Part print with two shaded views. Sizes in mm from the minimum x, y, z corner. Coordinates: 2 decimals unless noted, no trailing zeros. Loops run counter-clockwise (first coordinate to the right, second up) from the corner with the lowest first, then second, coordinate; pieces in that order, holes last.
(1) Slice it at B-B (z = 0.5). Give the cut face in (x, y).
(2) Slice it at A-A (x = 5.5). Give the cut face in (y, z), and give its area (3 significant figures).
(3) Flat gauge pin, fed straight in: P1, Ø0.6, axis at x = 0.5, z = 4.5, coming from the +Y side. Where does the tip first touch, or does it go through?
(4) Slice it at D-D (z = 2.5). Give the cut face in (x, y).
(5) Wall check: L1, parallel to Z at x = 5.75, y = 0.1; L2, parallel to X at y = 0.7, z = 1.6; L3, parallel to X at y = 0.6, z = 4.5. Give the ranges that are in metal, low to high.
(6) Slice it at C-C (y = 0.25). Give the cut face in (x, z).
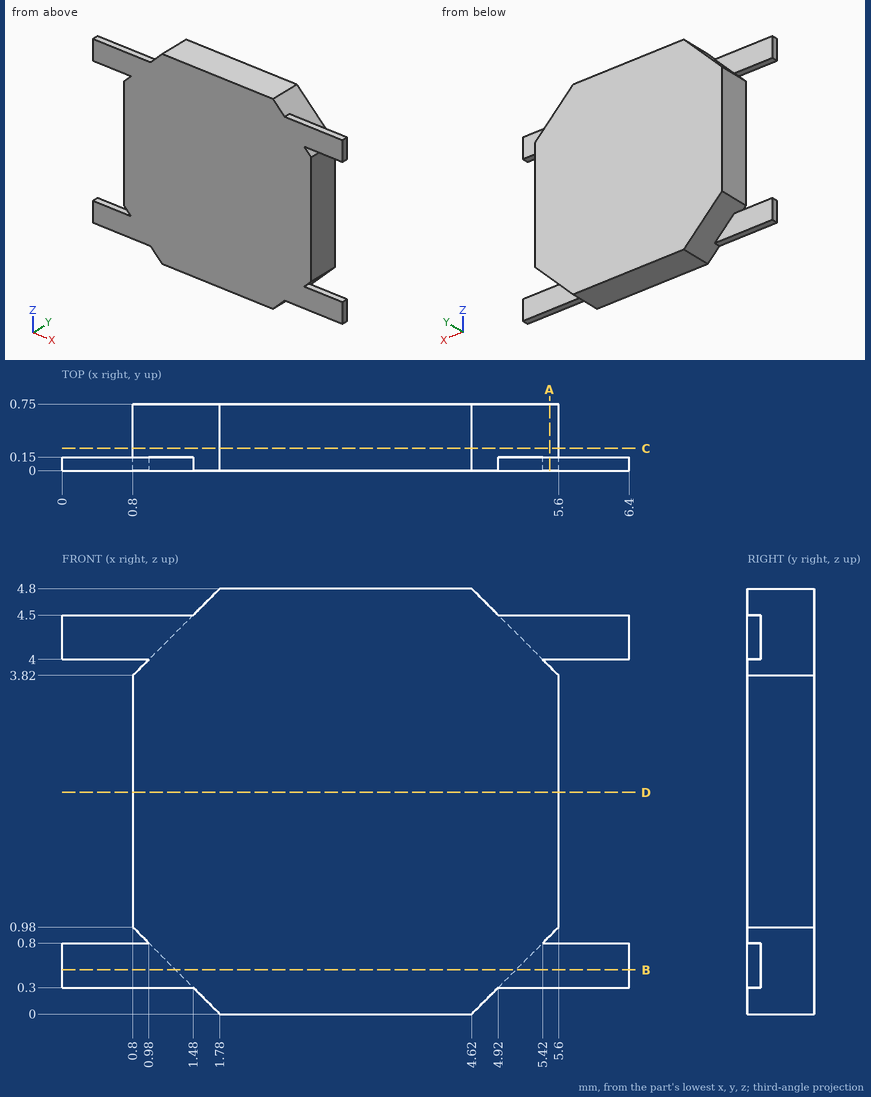
Response values:
1. outline: (0, 0) - (6.4, 0) - (6.4, 0.15) - (5.12, 0.15) - (5.12, 0.75) - (1.28, 0.75) - (1.28, 0.15) - (0, 0.15) - close
2. outline: (0, 0.3) - (0.15, 0.3) - (0.15, 0.8) - (0, 0.8) - close; (0, 0.88) - (0.75, 0.88) - (0.75, 3.92) - (0, 3.92) - close; (0, 4) - (0.15, 4) - (0.15, 4.5) - (0, 4.5) - close
2. area: 2.43 mm2
3. P1: stops at y = 0.15
4. outline: (0.8, 0) - (5.6, 0) - (5.6, 0.75) - (0.8, 0.75) - close
5. L1: z = 0.3 to 0.8, 4 to 4.5
5. L2: x = 0.8 to 5.6
5. L3: x = 1.48 to 4.92
6. outline: (0.8, 0.98) - (1.78, 0) - (4.62, 0) - (5.6, 0.98) - (5.6, 3.82) - (4.62, 4.8) - (1.78, 4.8) - (0.8, 3.82) - close
